Verification items for the finished model (mm, model axes). A direction names the side the tool comes from. Round coordinates to 2 decimals unless told otherwise and drop trailing zeros. Loops run counter-clockwise (first coordinate to the right, second up) from the corner with the lowest first, then second, coordinate; pieces in that order, holes last. Notation, with made-up numbers: M 77.5,-17.5 L 89.5,-17.5 A29 cw 89.5,5.5 Z; hole C 4,-25.5 d5. An arc over 180 degrees is marked long. One line per item, written item: value.
from build123d import *

# Parameters (mm, degrees)
SKETCH1_W           = 142.2
SKETCH1_H           = 136
BOSS_EXTRUDE1_DEPTH = 6
SKETCH2_W           = 142.2
SKETCH2_H           = 136
BOSS_EXTRUDE2_DEPTH = 3
CHAMFER1_SIZE       = 6
CHAMFER2_SIZE       = 4
SKETCH3_R           = 1.55
CUT_EXTRUDE1_DEPTH  = 2.3


with BuildPart() as part:
    # Sketch1 → Boss-Extrude1 (new body)
    with BuildSketch(Plane.XY):
        with Locations((-71.1, 68)):
            Rectangle(SKETCH1_W, SKETCH1_H)
        with BuildLine():
            ThreePointArc((-5, 9.5), (-7.121320344, 8.621320344), (-8, 6.5))
            Line((-8, 6.5), (-8, 5))
            Line((-8, 5), (-132.7, 5))
            Line((-132.7, 5), (-132.7, 6.5))
            ThreePointArc((-132.7, 6.5), (-133.578679656, 8.621320344), (-135.7, 9.5))
            Line((-135.7, 9.5), (-137.2, 9.5))
            Line((-137.2, 9.5), (-137.2, 126.5))
            Line((-137.2, 126.5), (-135.7, 126.5))
            ThreePointArc((-135.7, 126.5), (-133.578679656, 127.378679656), (-132.7, 129.5))
            Line((-132.7, 129.5), (-132.7, 131))
            Line((-132.7, 131), (-8, 131))
            Line((-8, 131), (-8, 129.5))
            ThreePointArc((-8, 129.5), (-7.121320344, 127.378679656), (-5, 126.5))
            Line((-5, 126.5), (-5, 9.5))
        make_face(mode=Mode.SUBTRACT)
    extrude(amount=BOSS_EXTRUDE1_DEPTH)

    # Sketch2 → Boss-Extrude2 (add)
    with BuildSketch(Plane.XY.offset(6)):
        with Locations((-71.1, 68)):
            Rectangle(SKETCH2_W, SKETCH2_H)
    extrude(amount=BOSS_EXTRUDE2_DEPTH)

    # Chamfer1
    chamfer1_edges = [part.edges().sort_by_distance(p)[0] for p in [
        (-142.2, 68, 9),
        (-71.1, 0, 9),
        (0, 68, 9),
        (-71.1, 136, 9),
    ]]
    chamfer(chamfer1_edges, length=CHAMFER1_SIZE)

    # Chamfer2
    # the kernel refuses this chamfer: 4 mm, written as the material it adds along each edge
    with BuildSketch(Plane(origin=(-142.986731952, 131, 6), x_dir=(0, 0.02749587661058907, -0.9996219169112965), z_dir=(1, 0, 0))) as chamfer2_piece_1_section:
        Polygon((CHAMFER2_SIZE * 0.999621916911, -CHAMFER2_SIZE * 0.0274958766106), (-CHAMFER2_SIZE * 0.0274958766106, -CHAMFER2_SIZE * 0.999621916911), (0, 0), align=None)
    chamfer2_piece_1 = extrude(amount=145.273463904, mode=Mode.PRIVATE)
    chamfer2_piece_1 = split(chamfer2_piece_1, bisect_by=Plane(origin=(-142.2, 127.973585933, 5.513207057), z_dir=(1, 0, 0)), keep=Keep.TOP, mode=Mode.PRIVATE)
    chamfer2_piece_1 = split(chamfer2_piece_1, bisect_by=Plane(origin=(0, 127.973585933, 5.513207057), z_dir=(-1, 0, 0)), keep=Keep.TOP, mode=Mode.PRIVATE)
    chamfer2_piece_1 = split(chamfer2_piece_1, bisect_by=Plane(origin=(-136.314439618, 127.973585933, 8.885560382), z_dir=(0.7071067811865476, 0, -0.7071067811865476)), keep=Keep.TOP, mode=Mode.PRIVATE)
    chamfer2_piece_1 = split(chamfer2_piece_1, bisect_by=Plane(origin=(-67.727646674, 127.973585933, 70.727646674), z_dir=(-0.7071067811865476, 0, -0.7071067811865476)), keep=Keep.TOP, mode=Mode.PRIVATE)
    add(chamfer2_piece_1)
    with BuildSketch(Plane(origin=(-5, 136.786731952, 6), x_dir=(0.02749587661058627, 0, -0.9996219169112968), z_dir=(0, -1, 0))) as chamfer2_piece_2_section:
        Polygon((CHAMFER2_SIZE * 0.999621916911, -CHAMFER2_SIZE * 0.0274958766106), (-CHAMFER2_SIZE * 0.0274958766106, -CHAMFER2_SIZE * 0.999621916911), (0, 0), align=None)
    chamfer2_piece_2 = extrude(amount=137.573463904, mode=Mode.PRIVATE)
    chamfer2_piece_2 = split(chamfer2_piece_2, bisect_by=Plane(origin=(-8.333333333, 5, 5.666666667), z_dir=(0, 1, 0)), keep=Keep.TOP, mode=Mode.PRIVATE)
    chamfer2_piece_2 = split(chamfer2_piece_2, bisect_by=Plane(origin=(-8.333333333, 131, 5.666666667), z_dir=(0, -1, 0)), keep=Keep.TOP, mode=Mode.PRIVATE)
    add(chamfer2_piece_2)
    with BuildSketch(Plane(origin=(2.286731952, 5, 6), x_dir=(0, -0.02749587661058627, -0.9996219169112968), z_dir=(-1, 0, 0))) as chamfer2_piece_3_section:
        Polygon((CHAMFER2_SIZE * 0.999621916911, -CHAMFER2_SIZE * 0.0274958766106), (-CHAMFER2_SIZE * 0.0274958766106, -CHAMFER2_SIZE * 0.999621916911), (0, 0), align=None)
    chamfer2_piece_3 = extrude(amount=145.273463904, mode=Mode.PRIVATE)
    chamfer2_piece_3 = split(chamfer2_piece_3, bisect_by=Plane(origin=(-142.2, 8.026414067, 5.513207057), z_dir=(1, 0, 0)), keep=Keep.TOP, mode=Mode.PRIVATE)
    chamfer2_piece_3 = split(chamfer2_piece_3, bisect_by=Plane(origin=(0, 8.026414067, 5.513207057), z_dir=(-1, 0, 0)), keep=Keep.TOP, mode=Mode.PRIVATE)
    chamfer2_piece_3 = split(chamfer2_piece_3, bisect_by=Plane(origin=(-73.722353326, 8.026414067, 71.477646674), z_dir=(0.7071067811865476, 0, -0.7071067811865476)), keep=Keep.TOP, mode=Mode.PRIVATE)
    chamfer2_piece_3 = split(chamfer2_piece_3, bisect_by=Plane(origin=(-5.135560382, 8.026414067, 8.135560382), z_dir=(-0.7071067811865476, 0, -0.7071067811865476)), keep=Keep.TOP, mode=Mode.PRIVATE)
    add(chamfer2_piece_3)
    with BuildSketch(Plane(origin=(-137.2, -0.786731952, 6), x_dir=(-0.02749587661058907, 0, -0.9996219169112965), z_dir=(0, 1, 0))) as chamfer2_piece_4_section:
        Polygon((CHAMFER2_SIZE * 0.999621916911, -CHAMFER2_SIZE * 0.0274958766106), (-CHAMFER2_SIZE * 0.0274958766106, -CHAMFER2_SIZE * 0.999621916911), (0, 0), align=None)
    chamfer2_piece_4 = extrude(amount=137.573463904, mode=Mode.PRIVATE)
    chamfer2_piece_4 = split(chamfer2_piece_4, bisect_by=Plane(origin=(-134.173585933, 0, 5.513207057), z_dir=(0, 1, 0)), keep=Keep.TOP, mode=Mode.PRIVATE)
    chamfer2_piece_4 = split(chamfer2_piece_4, bisect_by=Plane(origin=(-134.173585933, 5.885560382, 8.885560382), z_dir=(0, 0.7071067811865476, -0.7071067811865476)), keep=Keep.TOP, mode=Mode.PRIVATE)
    chamfer2_piece_4 = split(chamfer2_piece_4, bisect_by=Plane(origin=(-134.173585933, 136, 5.513207057), z_dir=(0, -1, 0)), keep=Keep.TOP, mode=Mode.PRIVATE)
    chamfer2_piece_4 = split(chamfer2_piece_4, bisect_by=Plane(origin=(-134.173585933, 71.372353326, 67.627646674), z_dir=(0, -0.7071067811865476, -0.7071067811865476)), keep=Keep.TOP, mode=Mode.PRIVATE)
    add(chamfer2_piece_4)

    # Sketch3 → Cut-Extrude1 (cut)
    with BuildSketch(Plane(origin=(0, 0, 0), x_dir=(-1, 0, 0), z_dir=(0, 0, -1))):
        with Locations((135.7, 129.5)):
            Circle(SKETCH3_R)
        with Locations((135.7, 6.5)):
            Circle(SKETCH3_R)
        with Locations((5, 6.5)):
            Circle(SKETCH3_R)
        with Locations((5, 129.5)):
            Circle(SKETCH3_R)
    extrude(amount=-CUT_EXTRUDE1_DEPTH, mode=Mode.SUBTRACT)


solid = part.part
(1) Sectioned sample at B-B on y = 37. Enter the section's corners in (x, z).
Completed:
outline: M -142.2,0 L -137.2,0 L -137.2,2 L -133.2,6 L -9,6 L -5,2 L -5,0 L 0,0 L 0,3 L -6,9 L -136.2,9 L -142.2,3 Z
(2) Mould release check, pull along X, two halves, no side actions. Record for faces 3 (the face through (-133.6, 127.36, 2.15)), 4 (the face through (-3, 69, 6)), 5 (the face through (-139.2, 69, 6)): +X half, -X half, draft (parallel to the pull), parting line (faces both ways), or undercut.
Completed:
face 3: undercut
face 4: +X half
face 5: -X half
(3) Sectioned sample at C-C on z = 7.5. Enter the section's corners in (x, y), and give its area (3 significant figures).
Completed:
outline: M -137.7,4.5 L -4.5,4.5 L -4.5,131.5 L -137.7,131.5 Z
area: 16,900 mm^2
(4) Thickness scan on L1, parallel to Y at x = -135.7, z = 0.6; L2, parallel to X at y = 129.5, z = 1.3; L3, parallel to Y at x = -43.5, z = 1.25. Record the ranges inside material, lowest first. Write a range as from..to.
Completed:
L1: y = 0..4.95, 8.05..9.5, 126.5..127.95, 131.05..136
L2: x = -142.2..-137.25, -134.15..-132.7, -8..-6.55, -3.45..0
L3: y = 0..5, 131..136
(5) Depth check by flat-ended pin: pin 1 Ø1.5 at (x, y) = (-86.5, 82.5) entering from -Z; pin 2 Ø0.9 at (x, y) = (-4.5, 6.5) entering from -Z; pin 3 Ø1.5 at (x, z) = (-115, 5.5) entering from +Y. Enter the tip coordinate at first touch or a pass-through.
Completed:
pin 1: stops at z = 6
pin 2: stops at z = 2.3
pin 3: stops at y = 134.25
(6) Tool access check on faces 1 (the face through (-135.364, 127.987, 1.134)), 2 (the face through (-72, 3, 6)). Record the directions out of +Z, -Z, +X, -X, +Y, -Y that give a thin tool (end or side, any length) a straight path to the whole face; none if there is none.
Completed:
face 1: -Z
face 2: +Z, +X, -X, -Y
(7) Sectioned sample at A-A on x = -128. Enter the section's corners in (y, z), and give its area (3 significant figures).
Completed:
outline: M 0,0 L 5,0 L 5,2 L 9,6 L 127,6 L 131,2 L 131,0 L 136,0 L 136,3 L 130,9 L 6,9 L 0,3 Z
area: 448 mm^2
